CAD build for the part. Positions are in the model's coordinates, mm. Face numbers are marked on the shaded views. A direction names the side the tool comes from. Give positions to 0.01 mm unless a question says otherwise; leave off trailing zeros. Loops run counter-clockwise (first coordinate to the right, second up) from the corner with the lowest first, then second, coordinate; pieces in that order, holes last.
Item 1: Saw through at A-A on z = 1304.5. Give the cut face in (x, y) (3 decimals).
Item 2: Drop flat-ended pins along their axis: P1, Ø8, axis at x = 831.5, y = 1096, coming from the -Z side; P2, Ø0.6, axis at x = 816.5, z = 1305, coming from the +Y side; P3, Ø1.8, axis at x = 792.65, y = 1097.59, coming from the +Z side; P4, Ø0.6, axis at x = 787, z = 1305, coming from the +Y side. Give the stop position or say it passes through.
Item 3: Saw through at D-D on y = 1086.5. Give the cut face in (x, z), plus the area to 3 significant figures.
Item 4: Probe probe 1 along X at (y, z) = (1094.5, 1316.5); probe 2 along Y at (x, z) = (807, 1311.5); probe 3 along X at (y, z) = (1114, 1312.5). List the from-to ranges inside material, lowest first.
Item 5: Which spindle directions (+Z, -Z, +X, -X, +Y, -Y) get a long thin tool onto all of the face, cutting with end or side? Do the marked faces 1, 2 and 3. Say none if no direction does.
Item 6: Mould opens along Y. For the marked faces 4, 5, 6 and 7 say: released by +Y, released by -Y, zero draft, split by the parting line, or undercut.
Item 7: Saw through at B-B on x = 830. Give the cut face in (y, z), plus the area to 3 significant figures.
Item 8: Saw through at C-C on z = 1308.5. Give the cut face in (x, y) (3 decimals).
from build123d import *

# Parameters (mm, degrees)
BOSS_EXTRUDE1_DEPTH = 15
BOSS_EXTRUDE2_DEPTH = 15
CUT_EXTRUDE1_DEPTH  = 14
SKETCH8_W           = 6.699223296
SKETCH8_H           = 4.721357371
SKETCH8_W_2         = 8.228893272
CUT_EXTRUDE7_DEPTH  = 3
SKETCH10_R          = 1.1
CUT_EXTRUDE9_DEPTH  = 15


with BuildPart() as part:
    # Sketch3 → Boss-Extrude1 (new body)
    with BuildSketch(Plane.XY.offset(1303.472903018)):
        with BuildLine():
            Line((839.650097305, 1097.589789038), (839.650097371, 1033.49652121))
            Line((839.650097371, 1033.49652121), (785.650097371, 1033.49652121))
            Line((785.650097371, 1033.49652121), (785.650097438, 1120.589789038))
            ThreePointArc((785.650097438, 1120.589789038), (787.114883847, 1124.124637961), (790.64973277, 1125.58942437))
            Line((790.64973277, 1125.58942437), (812.066461973, 1125.58942437))
            ThreePointArc((812.066461973, 1125.58942437), (815.601310896, 1124.124637961), (817.066097305, 1120.589789038))
            Line((817.066097305, 1120.589789038), (817.066097305, 1103.589789038))
            ThreePointArc((817.066097305, 1103.589789038), (817.35931084, 1102.882637905), (818.066461973, 1102.58942437))
            Line((818.066461973, 1102.58942437), (834.650461973, 1102.58942437))
            ThreePointArc((834.650461973, 1102.58942437), (838.185310896, 1101.124637961), (839.650097305, 1097.589789038))
        make_face()
        with BuildLine():
            Line((787.650097371, 1035.49652121), (787.650097371, 1120.589424436))
            ThreePointArc((787.650097371, 1120.589424436), (788.529097371, 1122.710424436), (790.650097371, 1123.589424436))
            Line((790.650097371, 1123.589424436), (812.066097371, 1123.589424436))
            ThreePointArc((812.066097371, 1123.589424436), (814.187097371, 1122.710424436), (815.066097371, 1120.589424436))
            Line((815.066097371, 1120.589424436), (815.066097371, 1103.589424436))
            ThreePointArc((815.066097371, 1103.589424436), (815.945097371, 1101.468424436), (818.066097371, 1100.589424436))
            Line((818.066097371, 1100.589424436), (834.650097371, 1100.589424436))
            ThreePointArc((834.650097371, 1100.589424436), (836.771097371, 1099.710424436), (837.650097371, 1097.589424436))
            Line((837.650097371, 1097.589424436), (837.650097371, 1035.49652121))
            Line((837.650097371, 1035.49652121), (787.650097371, 1035.49652121))
        make_face(mode=Mode.SUBTRACT)
    extrude(amount=BOSS_EXTRUDE1_DEPTH)

    # Sketch6 → Boss-Extrude2 (add)
    with BuildSketch(Plane.XY.offset(1303.472903018)):
        with BuildLine():
            Line((787.650097371, 1035.49652121), (837.650097371, 1035.49652121))
            Line((837.650097371, 1035.49652121), (837.650097371, 1097.589424436))
            ThreePointArc((837.650097371, 1097.589424436), (836.771097371, 1099.710424436), (834.650097371, 1100.589424436))
            Line((834.650097371, 1100.589424436), (818.066097371, 1100.589424436))
            ThreePointArc((818.066097371, 1100.589424436), (815.945097371, 1101.468424436), (815.066097371, 1103.589424436))
            Line((815.066097371, 1103.589424436), (815.066097371, 1120.589424436))
            ThreePointArc((815.066097371, 1120.589424436), (814.187097371, 1122.710424436), (812.066097371, 1123.589424436))
            Line((812.066097371, 1123.589424436), (790.650097371, 1123.589424436))
            ThreePointArc((790.650097371, 1123.589424436), (788.529097371, 1122.710424436), (787.650097371, 1120.589424436))
            Line((787.650097371, 1120.589424436), (787.650097371, 1035.49652121))
        make_face()
    extrude(amount=BOSS_EXTRUDE2_DEPTH)

    # Sketch6<2> → Cut-Extrude1 (cut)
    with BuildSketch(Plane.XY.offset(1303.472903018)):
        with BuildLine():
            Line((787.650097371, 1035.49652121), (837.650097371, 1035.49652121))
            Line((837.650097371, 1035.49652121), (837.650097371, 1097.589424436))
            ThreePointArc((837.650097371, 1097.589424436), (836.771097371, 1099.710424436), (834.650097371, 1100.589424436))
            Line((834.650097371, 1100.589424436), (818.066097371, 1100.589424436))
            ThreePointArc((818.066097371, 1100.589424436), (815.945097371, 1101.468424436), (815.066097371, 1103.589424436))
            Line((815.066097371, 1103.589424436), (815.066097371, 1120.589424436))
            ThreePointArc((815.066097371, 1120.589424436), (814.187097371, 1122.710424436), (812.066097371, 1123.589424436))
            Line((812.066097371, 1123.589424436), (790.650097371, 1123.589424436))
            ThreePointArc((790.650097371, 1123.589424436), (788.529097371, 1122.710424436), (787.650097371, 1120.589424436))
            Line((787.650097371, 1120.589424436), (787.650097371, 1035.49652121))
        make_face()
    extrude(amount=CUT_EXTRUDE1_DEPTH, mode=Mode.SUBTRACT)

    # Sketch8 → Cut-Extrude7 (cut)
    with BuildSketch(Plane.XY.offset(1303.472903018)):
        with Locations((788.177093813, 1120.255926572)):
            Rectangle(SKETCH8_W, SKETCH8_H)
        with Locations((813.958809837, 1120.255926572)):
            Rectangle(SKETCH8_W_2, SKETCH8_H)
    extrude(amount=CUT_EXTRUDE7_DEPTH, mode=Mode.SUBTRACT)

    # Sketch10 → Cut-Extrude9 (cut)
    with BuildSketch(Plane.XY.offset(1303.472903018)):
        with Locations((832.650097371, 1039.589424436)):
            Circle(SKETCH10_R)
        with Locations((792.650097371, 1039.589424436)):
            Circle(SKETCH10_R)
        with Locations((792.650097371, 1097.589424436)):
            Circle(SKETCH10_R)
        with Locations((812.650097371, 1097.589424436)):
            Circle(SKETCH10_R)
    extrude(amount=CUT_EXTRUDE9_DEPTH, mode=Mode.SUBTRACT)


solid = part.part
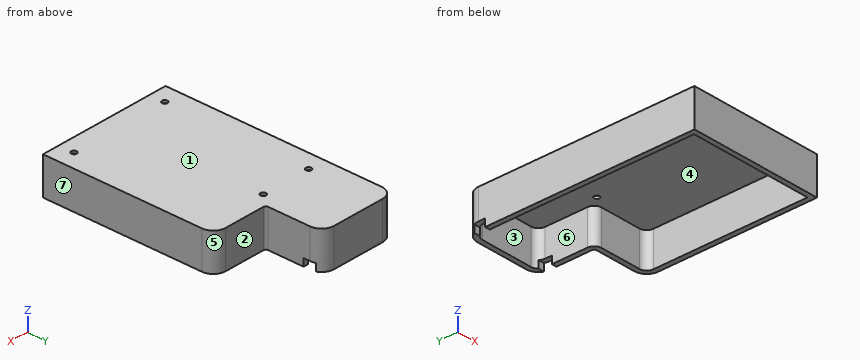
Results below:
1. outline: (785.65, 1033.497) - (839.65, 1033.497) - (839.65, 1097.59) arc R5.001 ccw to (834.65, 1102.589) - (818.066, 1102.589) arc R1.001 cw to (817.066, 1103.59) - (817.066, 1117.895) - (815.066, 1117.895) - (815.066, 1103.589) arc R3.001 ccw to (818.066, 1100.589) - (834.65, 1100.589) arc R3.001 cw to (837.65, 1097.589) - (837.65, 1035.497) - (787.65, 1035.497) - (787.65, 1117.895) - (785.65, 1117.895) - close; (786.08, 1122.617) - (788.439, 1122.617) arc R3.001 cw to (790.65, 1123.589) - (812.066, 1123.589) arc R3.001 cw to (814.277, 1122.617) - (816.636, 1122.617) arc R5.001 ccw to (812.066, 1125.589) - (790.65, 1125.589) arc R5.001 ccw to start
2. P1: stops at z = 1317.47
2. P2: stops at y = 1123.4
2. P3: passes through
2. P4: stops at y = 1124.3
3. outline: (785.65, 1303.47) - (787.65, 1303.47) - (787.65, 1317.47) - (837.65, 1317.47) - (837.65, 1303.47) - (839.65, 1303.47) - (839.65, 1318.47) - (785.65, 1318.47) - close
3. area: 110 mm2
4. probe 1: x = 785.65 to 787.65, 837.65 to 839.65
4. probe 2: y = 1033.5 to 1035.5, 1123.59 to 1125.59
4. probe 3: x = 785.65 to 787.65, 815.07 to 817.07
5. face 1: +Z, +X, -X, +Y, -Y
5. face 2: +Z, -Z, +X, +Y
5. face 3: -Z
6. face 4: undercut
6. face 5: released by +Y
6. face 6: undercut
6. face 7: zero draft
7. outline: (1033.5, 1303.47) - (1035.5, 1303.47) - (1035.5, 1317.47) - (1100.59, 1317.47) - (1100.59, 1303.47) - (1102.59, 1303.47) - (1102.59, 1318.47) - (1033.5, 1318.47) - close
7. area: 125 mm2
8. outline: (785.65, 1033.497) - (839.65, 1033.497) - (839.65, 1097.59) arc R5.001 ccw to (834.65, 1102.589) - (818.066, 1102.589) arc R1.001 cw to (817.066, 1103.59) - (817.066, 1120.59) arc R5.001 ccw to (812.066, 1125.589) - (790.65, 1125.589) arc R5.001 ccw to (785.65, 1120.59) - close; hole (787.65, 1035.497) - (837.65, 1035.497) - (837.65, 1097.589) arc R3.001 ccw to (834.65, 1100.589) - (818.066, 1100.589) arc R3.001 cw to (815.066, 1103.589) - (815.066, 1120.589) arc R3.001 ccw to (812.066, 1123.589) - (790.65, 1123.589) arc R3.001 ccw to (787.65, 1120.589) - close
